```python
from build123d import *

# Parameters (mm, degrees)
F0_R     = 38.1
F0_R_2   = 31.75
F1_DEPTH = 6.35
F2_R     = 2.54
F3_DEPTH = 69.85
F4_R     = 38.1
F4_R_2   = 31.75
F4_R_3   = 2.54
F5_DEPTH = 6.35


with BuildPart() as f1:
    # F0 (on Top) → F1 (new body)
    with BuildSketch(Plane.XY):
        Circle(F0_R)
        Circle(F0_R_2, mode=Mode.SUBTRACT)
    extrude(amount=F1_DEPTH)

    # F2 (on face) → F3 (join)
    with BuildSketch(Plane.XY.offset(6.35)):
        with Locations((24.695704, 24.695704)):
            Circle(F2_R)
        with Locations((34.925, 0)):
            Circle(F2_R)
        with Locations((24.695704, -24.695704)):
            Circle(F2_R)
        with Locations((0, -34.925)):
            Circle(F2_R)
        with Locations((-24.695704, -24.695704)):
            Circle(F2_R)
        with Locations((-34.925, 0)):
            Circle(F2_R)
        with Locations((-24.695704, 24.695704)):
            Circle(F2_R)
        with Locations((0, 34.925)):
            Circle(F2_R)
    extrude(amount=F3_DEPTH)

    # F4 (on face) → F5 (join)
    with BuildSketch(Plane.XY.offset(76.2)):
        Circle(F4_R)
        Circle(F4_R_2, mode=Mode.SUBTRACT)
        with Locations((0, 34.925)):
            Circle(F4_R_3, mode=Mode.SUBTRACT)
        with Locations((0, 34.925)):
            Circle(F4_R_3)
    extrude(amount=F5_DEPTH)


solid = f1.part
```
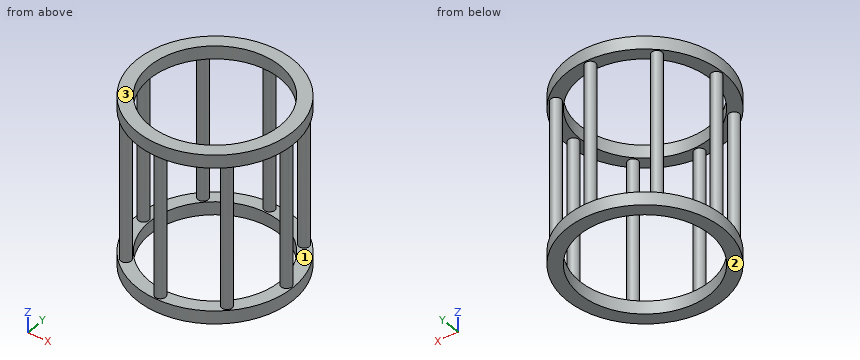
For this review, take the finished solid that the model builds, in its own axes (mm). Face numbers are marked on the shaded views. Give positions to 0.01 mm unless a question says otherwise; leave off trailing zeros. Order: outer loops, then holes, each group sorted by start corner. A loop starts at its lowest first (then second) coordinate and runs counter-clockwise, first axis right, second up.
1) Take a section at D-D (x = 19). Give the boundary of the cut face in (y, z).
2) Take a section at A-A (x = 0). Give the boundary of the cut face in (y, z) (3 decimals), then the cut area to 3 significant figures.
3) The part is to be moulded in two halves that separate along Z. For the marked faces 1, 2 and 3, say which applies: released by +Z, released by -Z, zero draft, split by the parting line, or undercut.
4) Take a section at C-C (y = 11.5). Give the boundary of the cut face in (x, z), then the cut area to 3 significant figures.
5) Insertion check: pin 1 (10 mm diameter, centred on y = -30, z = 42.5, fed in from -X); pin 2 (6 mm diameter, centred on y = -2, z = 43, fed in from -X) (3 decimals); pin 3 (8 mm diameter, centred on x = -21, z = 16.5, fed in from +Y). Each pin has a flat end and moves straight along its axis. Give the tip position at first contact, or say it passes through.
6) Wall thickness on line 1 (Y direction, x = 0, z = 78); line 2 (X direction, y = -10.5, z = 4); line 3 (X direction, y = -21, z = 6): over which ranges is each line inside the solid? List them lowest first.
Derived:
1. outline: (-33.02, 0) - (-25.44, 0) - (-25.44, 6.35) - (-33.02, 6.35) - close; (-33.02, 76.2) - (-25.44, 76.2) - (-25.44, 82.55) - (-33.02, 82.55) - close; (25.44, 0) - (33.02, 0) - (33.02, 6.35) - (25.44, 6.35) - close; (25.44, 76.2) - (33.02, 76.2) - (33.02, 82.55) - (25.44, 82.55) - close
2. outline: (-38.1, 0) - (-31.75, 0) - (-31.75, 6.35) - (-32.385, 6.35) - (-32.385, 76.2) - (-31.75, 76.2) - (-31.75, 82.55) - (-38.1, 82.55) - (-38.1, 76.2) - (-37.465, 76.2) - (-37.465, 6.35) - (-38.1, 6.35) - close; (31.75, 0) - (38.1, 0) - (38.1, 6.35) - (37.465, 6.35) - (37.465, 76.2) - (38.1, 76.2) - (38.1, 82.55) - (31.75, 82.55) - (31.75, 76.2) - (32.385, 76.2) - (32.385, 6.35) - (31.75, 6.35) - close
2. area: 871 mm2
3. face 1: undercut
3. face 2: released by -Z
3. face 3: released by +Z
4. outline: (-36.32, 0) - (-29.59, 0) - (-29.59, 6.35) - (-36.32, 6.35) - close; (-36.32, 76.2) - (-29.59, 76.2) - (-29.59, 82.55) - (-36.32, 82.55) - close; (29.59, 0) - (36.32, 0) - (36.32, 6.35) - (29.59, 6.35) - close; (29.59, 76.2) - (36.32, 76.2) - (36.32, 82.55) - (29.59, 82.55) - close
4. area: 171 mm2
5. pin 1: stops at x = -27.22
5. pin 2: stops at x = -37.465
5. pin 3: stops at y = 27.24
6. line 1: y = -38.1 to -31.75, 31.75 to 38.1
6. line 2: x = -36.62 to -29.96, 29.96 to 36.62
6. line 3: x = -31.79 to -23.81, 23.81 to 31.79
